Autodesk Inventor part; units mm, degrees
ref_plane "YZ Plane" through (0, 0, 0) normal (1, 0, 0) x (0, 1, 0)
ref_plane "XZ Plane" through (0, 0, 0) normal (0, 1, 0) x (-1, 0, 0)
ref_plane "XY Plane" through (0, 0, 0) normal (0, 0, 1) x (1, 0, 0)
sketch "Sketch1" plane through (0, 0, 0) normal (0, 0, 1) x (1, 0, 0)
  line L0 (-12.7, -25.4) -> (12.7, -25.4)
  line L1 (12.7, -25.4) -> (12.7, 25.4)
  line L2 (12.7, 25.4) -> (-12.7, 25.4)
  line L3 (-12.7, 25.4) -> (-12.7, -25.4)
  line L4 (-12.7, -25.4) -> (12.7, 25.4) construction
  line L5 (12.7, -25.4) -> (-12.7, 25.4) construction
  line L6 (-10.16, -22.86) -> (10.16, -22.86)
  line L7 (10.16, -22.86) -> (10.16, 22.86)
  line L8 (10.16, 22.86) -> (-10.16, 22.86)
  line L9 (-10.16, 22.86) -> (-10.16, -22.86)
  line L10 (-10.16, -22.86) -> (10.16, 22.86) construction
  line L11 (10.16, -22.86) -> (-10.16, 22.86) construction
  point P0 (0, 0)
  dimension "d0" = 25.4
  dimension "d1" = 50.8
  dimension "d2" = 20.32
  dimension "d3" = 45.72
extrude "Extrusion1" add sketch "Sketch1" along normal mid plane 508
sketch "Sketch2" plane through (-12.7, 25.4, 254) normal (0, 1, 0) x (1, 0, 0)
  line L0 (0, 508) -> (0, 0)
  line L1 (25.4, 0) -> (0, 0)
  point P0 (12.7, 254)
  point P1 (12.7, 12.7)
  dimension "d6" = 12.7
  dimension "d7" = 12.7
hole "Hole1" at (0, 25.4, 241.3) direction (0, -1, 0) diameter 4.1402 end through all
pattern_linear "Rectangular Pattern1" count 20 spacing 25.4 along (0, 0, -1) of "Hole1"
properties part number "Stationary_Horizontal_extender"
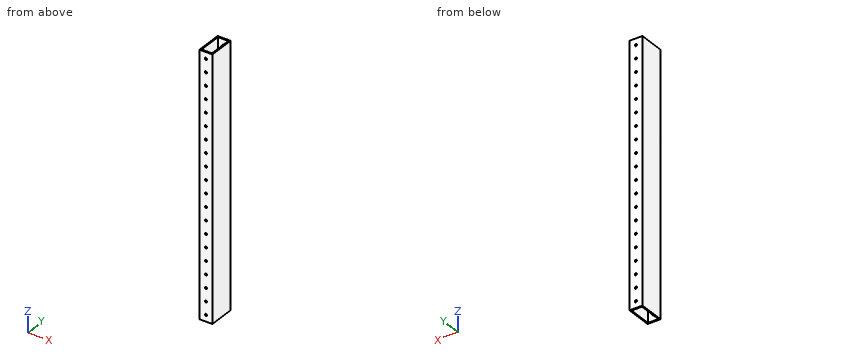
Input: part model. Units: mm. Frame: model coordinates. Coordinates: 2 decimals unless noted, no trailing zeros. Loops run counter-clockwise (first coordinate to the right, second up) from the corner with the lowest first, then second, coordinate; pieces in that order, holes last.
(1) Section B-B on z = 150.5. Return the cut outline in (x, y).
(2) Section A-A on y = -11.5. Return the cut outline in (x, z).
(3) First-contact query: pin 1 Ø5 at (x, z) = (0, -165.1) entering from -Y; pin 2 Ø3.5 at (x, z) = (0, -241.3) entering from +Y. Flat tips, straight axial feed; report the tip coordinate or a pass-through.
(4) Material intervals for probe 1 along Y at (x, z) = (-3.5, 0); probe 2 along X at (y, z) = (19, 175.5); probe 3 along X at (y, z) = (-23.7, -139.7), sorted ascending.
Data:
1. outline: (-12.7, -25.4) - (12.7, -25.4) - (12.7, 25.4) - (-12.7, 25.4) - close; hole (-10.16, -22.86) - (10.16, -22.86) - (10.16, 22.86) - (-10.16, 22.86) - close
2. outline: (-12.7, -254) - (-10.16, -254) - (-10.16, 254) - (-12.7, 254) - close; (10.16, -254) - (12.7, -254) - (12.7, 254) - (10.16, 254) - close
3. pin 1: stops at y = -25.4
3. pin 2: passes through
4. probe 1: y = -25.4 to -22.86, 22.86 to 25.4
4. probe 2: x = -12.7 to -10.16, 10.16 to 12.7
4. probe 3: x = -12.7 to -2.07, 2.07 to 12.7
